Model file for the job. Use its own axes, mm. Face numbers are marked on the shaded views. A direction names the side the tool comes from. Coordinates: 2 decimals unless noted, no trailing zeros. Loops run counter-clockwise (first coordinate to the right, second up) from the corner with the lowest first, then second, coordinate; pieces in that order, holes last. Notation, with made-up numbers: (50.5, 80) -> (55.5, 80) arc R6 cw to (55.5, 89) -> close; hole circle Ø8 at (16.5, -38). An arc over 180 degrees is marked (long way). Use one line per item in the form item = value.
```python
from build123d import *

# Parameters (mm, degrees)
PAD_DEPTH       = 5
SKETCH001_R     = 5
PAD001_DEPTH    = 12
PAD002_DEPTH    = 10
SKETCH003_W     = 40
SKETCH003_H     = 10
POCKET_DEPTH    = 40
POCKET001_DEPTH = 40
SKETCH005_R     = 5
POCKET002_DEPTH = 30


with BuildPart() as part:
    # Sketch → Pad (new body, symmetric)
    with BuildSketch(Plane.XY):
        with BuildLine():
            ThreePointArc((0, 20), (-20, 0), (0, -20))
            Line((0, -20), (119.999969, -20))
            ThreePointArc((119.999969, -20), (140, -1.6e-05), (120, 20))
            Line((0, 20), (120, 20))
        make_face()
    extrude(amount=PAD_DEPTH, both=True)

    # Sketch001 (on Face6 of Pad) → Pad001 (join)
    with BuildSketch(Plane.XY.offset(5)):
        Circle(SKETCH001_R)
    pad001 = extrude(amount=PAD001_DEPTH)

    # Sketch002 (on Face5 of Pad001) → Pad002 (join)
    with BuildSketch(Plane.XY.offset(5)):
        with BuildLine():
            Line((90, 20), (119.999998, 20))
            ThreePointArc((120.000041, -20), (140, 2.1e-05), (119.999998, 20))
            Line((120.000041, -20), (90, -20))
            Line((90, -20), (90, 20))
        make_face()
    pad002 = extrude(amount=PAD002_DEPTH)

    # Mirrored: Pad002 across XY
    add(pad002.mirror(Plane.XY))

    # Mirrored001: Pad001 across XY
    add(pad001.mirror(Plane.XY))

    # Sketch003 (on Face3 of Mirrored001) → Pocket (cut, symmetric)
    with BuildSketch(Plane.XZ.offset(20)):
        with Locations((120, 0)):
            Rectangle(SKETCH003_W, SKETCH003_H)
    extrude(amount=POCKET_DEPTH, both=True, mode=Mode.SUBTRACT)

    # Sketch004 (on Face10 of Pocket) → Pocket001 (cut)
    with BuildSketch(Plane.XZ.offset(20)):
        Polygon((90, 15), (90, 5), (100, 15), align=None)
    pocket001 = extrude(amount=-POCKET001_DEPTH, mode=Mode.SUBTRACT)

    # Mirrored002: Pocket001 across XY
    add(pocket001.mirror(Plane.XY), mode=Mode.SUBTRACT)

    # Sketch005 (on Face20 of Mirrored002) → Pocket002 (cut)
    with BuildSketch(Plane.XY.offset(15)):
        with Locations((120, 0)):
            Circle(SKETCH005_R)
    extrude(amount=-POCKET002_DEPTH, mode=Mode.SUBTRACT)


solid = part.part
```
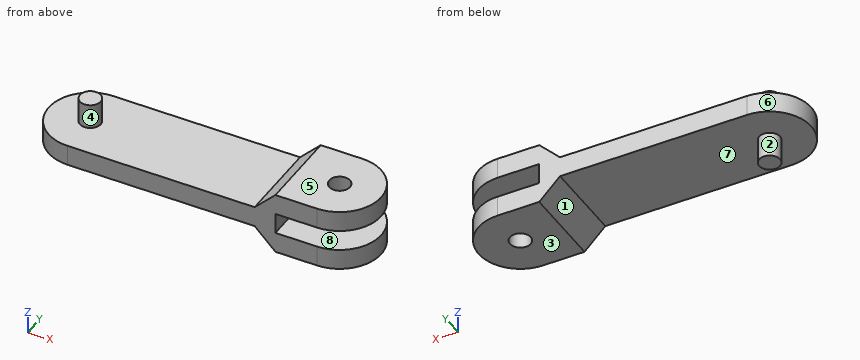
Q1. Band-saw the part on D-D, the plane y = -15.5. Write the cut outline in (x, z), and give its area (3 significant figures).
Result:
outline = (-12.64, -5) -> (90, -5) -> (100, -15) -> (132.64, -15) -> (132.64, -5) -> (100, -5) -> (100, 5) -> (132.64, 5) -> (132.64, 15) -> (100, 15) -> (90, 5) -> (-12.64, 5) -> close
area = 1,880 mm2
Q2. Band-saw the part on A-A, the plane x = 107. Write the cut outline in (y, z).
Result:
outline = (-20, -15) -> (20, -15) -> (20, -5) -> (-20, -5) -> close; (-20, 5) -> (20, 5) -> (20, 15) -> (-20, 15) -> close
Q3. Wall check: line 1 along Z through (x, y) = (102.5, -11.5); line 2 along X through (y, z) = (0.5, 7); line 3 along Y through (x, z) = (120, -7.5). Give the ranges that are in metal, low to high.
Result:
line_1 = -15 to -5, 5 to 15
line_2 = -4.97 to 4.97, 92 to 115.03, 124.97 to 139.99
line_3 = -20 to -5, 5 to 20
Q4. Mould opens along X. For the marked faces 6, 7 and 8 say: released by +X, released by -X, zero draft, split by the parting line, or undercut.
Result:
face_6 = released by -X
face_7 = undercut
face_8 = zero draft
Q5. Pin check, flat tips, straight feed: pin 1 Ø10 at (x, y) = (52, 14) entering from +Z; pin 2 Ø8 at (y, z) = (-6.5, -3.5) entering from +X; pin 3 Ø1.5 at (x, y) = (93, 12) entering from +Z. Stop position of each tip, or through.
Result:
pin_1 = 5
pin_2 = 139.8
pin_3 = 8.75
Q6. Which spindle directions (+Z, -Z, +X, -X, +Y, -Y) get a long thin tool onto all of the face, cutting with end or side? Do the marked faces 1, 2, 3, 4 and 5. Say none if no direction does.
Result:
face_1 = -Z, +Y, -Y
face_2 = -Z
face_3 = -Z, +X, +Y, -Y
face_4 = +Z
face_5 = +Z, +X, +Y, -Y
Q7. Band-saw the part on B-B, the plane y = 0. Write the cut outline in (x, z).
Result:
outline = (-20, -5) -> (-5, -5) -> (-5, -17) -> (5, -17) -> (5, -5) -> (90, -5) -> (100, -15) -> (115, -15) -> (115, -5) -> (100, -5) -> (100, 5) -> (115, 5) -> (115, 15) -> (100, 15) -> (90, 5) -> (5, 5) -> (5, 17) -> (-5, 17) -> (-5, 5) -> (-20, 5) -> close; (125, -15) -> (140, -15) -> (140, -5) -> (125, -5) -> close; (125, 5) -> (140, 5) -> (140, 15) -> (125, 15) -> close
Q8. Band-saw the part on C-C, the plane z = 10.5. Write the cut outline in (x, y), and give its area (3 significant figures).
Result:
outline = circle Ø10 at (0, 0); (95.5, -20) -> (120, -20) arc R20 ccw to (120, 20) -> (95.5, 20) -> close; hole circle Ø10 at (120, 0)
area = 1,610 mm2
